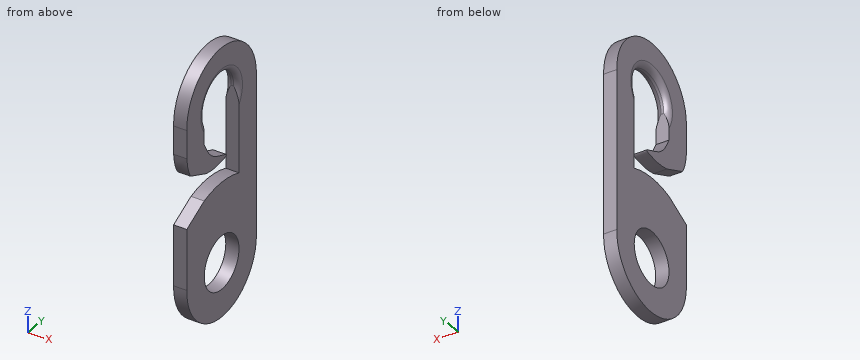
from build123d import *

# Parameters (mm, degrees)
F0_R        = 6.35
F1_DEPTH    = 3.175
F2_T1_DEPTH = 3.2744561413
F2_T4_ANGLE = 281.2740332969
F2_T6_ANGLE = 281.2740332969


# Not quite as in the source:
# - a fillet or chamfer that OpenCascade refuses, or shapes differently, is made with other operations: its cross-section is extruded or revolved along the edge and cut away or added


with BuildPart() as f1:
    # F0 (on Right) → F1 (new body)
    with BuildSketch(Plane.YZ):
        with BuildLine():
            Line((6.35, 19.05), (6.35, -1.0894877579))
            ThreePointArc((6.35, -1.0894877579), (0, 0), (-6.35, -1.0894877579))
            add(Edge.make_bspline(
                [(-6.35, -1.0894877579), (-8.4666666667, -2.2262237484), (-10.5833333333, -3.3629597389), (-12.7, -4.4996957295)],
                knots=[0, 0, 0, 0, 7.2077748584, 7.2077748584, 7.2077748584, 7.2077748584], degree=3))
            Line((-12.7, -4.4996957295), (-12.7, -18.9636734782))
            ThreePointArc((-12.7, -18.9636734782), (0, -31.9618793041), (12.7, -18.9636734782))
            Line((12.7, -18.9636734782), (12.7, 18.9636734782))
            ThreePointArc((12.7, 18.9636734782), (0, 31.9618793041), (-12.7, 18.9636734782))
            Line((-12.7, 18.9636734782), (-12.7, 12.2655965388))
            add(Edge.make_bspline(
                [(-12.7, 12.2655965388), (-12.5460680886, 10.8009133444), (-12.3921361771, 9.3362301501), (-11.3107701764, 7.4001117609)],
                knots=[0, 0, 0, 0, 0.2800418332, 0.2800418332, 0.2800418332, 0.2800418332], degree=3))
            add(Edge.make_bspline(
                [(-5.5794117662, 5), (-7.4898645696, 5.8000372536), (-9.400317373, 6.6000745073), (-11.3107701764, 7.4001117609)],
                knots=[0, 0, 0, 0, 6.2136145432, 6.2136145432, 6.2136145432, 6.2136145432], degree=3))
            add(Edge.make_bspline(
                [(-5.5794117662, 5), (-5.5956610435, 6.8858619014), (-5.9728305218, 9.5757292201), (-6.35, 12.2655965388)],
                knots=[0.7796078974, 0.7796078974, 0.7796078974, 0.7796078974, 1, 1, 1, 1], degree=3))
            Line((-6.35, 12.2655965388), (-6.35, 19.05))
            ThreePointArc((-6.35, 19.05), (0, 25.6118793041), (6.35, 19.05))
        make_face()
        with Locations((0, -19.05)):
            Circle(F0_R, mode=Mode.SUBTRACT)
        with BuildLine():
            add(Edge.make_bspline(
                [(-5.5794117662, 5), (-3.2248544463, 4.5091538123), (-0.6564824192, 4.8391769932), (3.3416252338, 5.6570567656), (-3.834716226, 7.1463236629), (-5.3129484548, 10.1981831131), (-6.35, 12.2655965388)],
                knots=[0, 0, 0, 0, 0.2814277691, 0.4456370567, 0.7068849416, 1, 1, 1, 1], degree=3))
            add(Edge.make_bspline(
                [(-5.5794117662, 5), (-5.5956610435, 6.8858619014), (-5.9728305218, 9.5757292201), (-6.35, 12.2655965388)],
                knots=[0.7796078974, 0.7796078974, 0.7796078974, 0.7796078974, 1, 1, 1, 1], degree=3))
        make_face()
    extrude(amount=F1_DEPTH)

    # F2: fillet of radius 1.27 on 4 edges, made by hand

    # F2_s2 → F2_t1 (cut)
    with BuildSketch(Plane.YZ.offset(-0.0497280707)):
        with BuildLine():
            ThreePointArc((-6.3505698659, 19.0681499948), (-6.3501424745, 19.0491315173), (-6.35, 19.0301087717))
            Line((-6.35, 19.0301087717), (-6.35, 19.05))
            ThreePointArc((-6.35, 19.05), (-6.3502914173, 19.0590747938), (-6.3505698659, 19.0681499948))
        make_face()
        with BuildLine():
            ThreePointArc((6.3505698659, 19.0681499948), (6.3501424745, 19.0491315173), (6.35, 19.0301087717))
            Line((6.35, 19.0301087717), (6.35, 19.05))
            ThreePointArc((6.35, 19.05), (6.3502914173, 19.0590747938), (6.3505698659, 19.0681499948))
        make_face()
    extrude(amount=F2_T1_DEPTH, mode=Mode.SUBTRACT)

    # F2_s3 → F2_t4 (revolve, cut)
    with BuildSketch(Plane(origin=(0, -9.4434175303, 7.7466985416), x_dir=(1, 0, 0), z_dir=(0, 0.7731434877, -0.6342311467))):
        with BuildLine():
            ThreePointArc((1.27, -8.5361310993), (0.3719743879, -8.1641567114), (0, -7.2661310993))
            Line((0, -7.2661310993), (0, -8.5361310993))
            Line((0, -8.5361310993), (1.27, -8.5361310993))
        make_face()
    revolve(axis=Axis((0, 0, 19.2584585737), (-1, 0, 0)), revolution_arc=F2_T4_ANGLE, mode=Mode.SUBTRACT)

    # F2_s5 → F2_t6 (revolve, cut)
    with BuildSketch(Plane(origin=(0, -9.4434175303, 7.7466985416), x_dir=(1, 0, 0), z_dir=(0, 0.7731434877, -0.6342311467))):
        with BuildLine():
            ThreePointArc((1.905, -8.5361310993), (2.8030256121, -8.1641567114), (3.175, -7.2661310993))
            Line((3.175, -7.2661310993), (3.175, -8.5361310993))
            Line((3.175, -8.5361310993), (1.905, -8.5361310993))
        make_face()
    revolve(axis=Axis((3.175, 0, 19.2584585737), (-1, 0, 0)), revolution_arc=F2_T6_ANGLE, mode=Mode.SUBTRACT)


solid = f1.part
The model under review builds one solid part; all positions refer to its coordinate system, in mm. Give positions to 0.01 mm unless a question says otherwise; leave off trailing zeros. Write each loop counter-clockwise with the first axis right and the second up, starting at its lowest first coordinate (ties: lowest second). Pieces come first, ordered by that corner, then holes.
1. For P1, Ø1, axis at x = 1, y = -4, coming from the +Z side; P2, Ø1, axis at x = 1.5, z = -12.5, coming from the -Y side; P3, Ø1, axis at x = 2, z = -22, coming from the +Y side, all flat-tipped, find the tip position at first contact; note any pin that passes through.
2. Add section A-A, the plane z = -22.5. Write out the cut boundary in (x, y) (3 decimals).
3. Add section B-B, the plane y = 0. Count the separate pieces of the cut face and the enclosed holes in it, plus the area to 3 significant figures.
4. Add section C-C, the plane z = 4. Write out the cut boundary in (x, y) (3 decimals), plus the area to 3 significant figures.
5. Add section D-D, the plane y = 9.5. Write out the cut boundary in (x, z) (3 decimals).
6. Wall thickness on L1, parallel to Z at x = 1.4, y = 3; L2, parallel to Z at x = 1.45, y = 0; L3, parallel to Z at x = 0.4, y = -3: over which ranges is each line inside the solid? List them lowest first.
Worked answers:
1. P1: stops at z = 31.47
1. P2: stops at y = -12.7
1. P3: stops at y = 12.5
2. outline: (0, -12.283) - (3.175, -12.283) - (3.175, -5.331) - (0, -5.331) - close; (0, 5.331) - (3.175, 5.331) - (3.175, 12.283) - (0, 12.283) - close
3. separate pieces: 4
3. enclosed holes: 0
3. area: 85.1 mm2
4. outline: (0, 6.35) - (3.175, 6.35) - (3.175, 12.7) - (0, 12.7) - close
4. area: 20.2 mm2
5. outline: (0, -27.692) - (3.175, -27.692) - (3.175, 27.692) - (0, 27.692) - close
6. L1: z = -31.6 to -24.65, -13.45 to -0.24, 24.86 to 31.6
6. L2: z = -31.96 to -25.4, -12.7 to 0, 5 to 6.41, 25.61 to 31.96
6. L3: z = -31.6 to -24.65, -13.45 to -0.24, 4.71 to 7.74, 25.25 to 31.6
